Build history of the part. All positions in model axes, mm. Face numbers are marked on the shaded views. A direction names the side the tool comes from. Coordinates: 2 decimals unless noted, no trailing zeros. Loops run counter-clockwise (first coordinate to the right, second up) from the corner with the lowest first, then second, coordinate; pieces in that order, holes last.
Item 1: Cut at C-C (x = -0.25). List the corners of the cut face in (y, z), and give its area (3 significant figures).
Item 2: Drill centre lines: line 1 along X through (y, z) = (-0.25, 4); line 2 along Y through (x, z) = (8.48, 3.75); line 3 along X through (y, z) = (-0.5, 2). Where is each one in solid material? Low to high.
Item 3: Cut at A-A (z = 1.5). List the corners of the cut face in (x, y) (3 decimals), and give its area (3 significant figures).
Item 4: 3-axis set-ups, long thin cutter, end or side, ignore diameter. For the marked faces 1 and 2: which of +Z, -Z, +X, -X, +Y, -Y reach the whole face in a straight line?
Item 5: Flat gauge pin, fed straight in: pin 1 (4 mm diameter, centred on x = 3, y = 1, fed in from +Z). Where does the tip first touch, or does it go through?
Item 6: Cut at D-D (y = -2). List the corners of the cut face in (x, z), and give its area (3 significant figures).
Item 7: Cut at B-B (y = 0). List the corners of the cut face in (x, z).
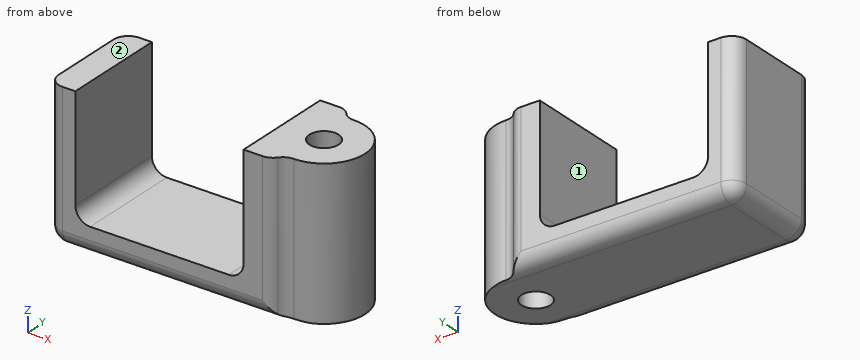
from build123d import *

# Parameters (mm, degrees)
F0_W         = 1.85
F0_H         = 7
F0_W_2       = 11.3
F1_DEPTH     = 1.85
F2_DEPTH     = 8
F3_T1_DEPTH  = 9.85
F3_T3_DEPTH  = 9.85
F3_T5_DEPTH  = 7
F3_T7_DEPTH  = 7
F3_T9_DEPTH  = 12
F4_T1_DEPTH  = 11.35
F4_T3_DEPTH  = 16.5
F4_T5_DEPTH  = 12.8150682373
F4_T8_ANGLE  = 90.0000000053
F4_T10_ANGLE = 90.0000000053


# Not quite as in the source:
# - a fillet or chamfer that OpenCascade refuses, or shapes differently, is made with other operations: its cross-section is extruded or revolved along the edge and cut away or added


with BuildPart() as f1:
    # F0 (on Top) → F1 (new body)
    with BuildSketch(Plane.XY):
        with Locations((-6.575, 0)):
            Rectangle(F0_W, F0_H)
        Rectangle(F0_W_2, F0_H)
        with BuildLine():
            Line((7.5, 0), (7.5, 2.5694551952))
            ThreePointArc((7.5, 2.5694551952), (5.73, 0), (7.5, -2.5694551952))
            Line((7.5, -2.5694551952), (7.5, 0))
        make_face()
        with BuildLine():
            Line((7.5, 2.5694551952), (7.5, 3.5))
            Line((7.5, 3.5), (5.65, 3.5))
            Line((5.65, 3.5), (5.65, -3.5))
            Line((5.65, -3.5), (7.5, -3.5))
            Line((7.5, -3.5), (7.5, -2.5694551952))
            ThreePointArc((7.5, -2.5694551952), (5.73, 0), (7.5, 2.5694551952))
        make_face()
        with BuildLine():
            ThreePointArc((11.23, 0), (10.0400480762, 2.2646743695), (7.5, 2.5694551952))
            Line((7.5, 2.5694551952), (7.5, 0))
            Line((7.5, 0), (7.5, -2.5694551952))
            ThreePointArc((7.5, -2.5694551952), (10.0400480762, -2.2646743695), (11.23, 0))
        make_face()
        with BuildLine():
            ThreePointArc((9.46, 0), (8.48, -0.98), (7.5, 0))
            ThreePointArc((7.5, 0), (8.48, 0.98), (9.46, 0))
        make_face(mode=Mode.SUBTRACT)
    extrude(amount=-F1_DEPTH)

    # F0 (on Top) → F2 (join)
    with BuildSketch(Plane.XY):
        with Locations((-6.575, 0)):
            Rectangle(F0_W, F0_H)
        with BuildLine():
            Line((7.5, 2.5694551952), (7.5, 3.5))
            Line((7.5, 3.5), (5.65, 3.5))
            Line((5.65, 3.5), (5.65, -3.5))
            Line((5.65, -3.5), (7.5, -3.5))
            Line((7.5, -3.5), (7.5, -2.5694551952))
            ThreePointArc((7.5, -2.5694551952), (5.73, 0), (7.5, 2.5694551952))
        make_face()
        with BuildLine():
            Line((7.5, 0), (7.5, 2.5694551952))
            ThreePointArc((7.5, 2.5694551952), (5.73, 0), (7.5, -2.5694551952))
            Line((7.5, -2.5694551952), (7.5, 0))
        make_face()
        with BuildLine():
            ThreePointArc((11.23, 0), (10.0400480762, 2.2646743695), (7.5, 2.5694551952))
            Line((7.5, 2.5694551952), (7.5, 0))
            Line((7.5, 0), (7.5, -2.5694551952))
            ThreePointArc((7.5, -2.5694551952), (10.0400480762, -2.2646743695), (11.23, 0))
        make_face()
        with BuildLine():
            ThreePointArc((9.46, 0), (8.48, -0.98), (7.5, 0))
            ThreePointArc((7.5, 0), (8.48, 0.98), (9.46, 0))
        make_face(mode=Mode.SUBTRACT)
    extrude(amount=F2_DEPTH)

    # F3: fillet of radius 1 on 5 edges, made by hand

    # F3_s2 → F3_t1 (join)
    with BuildSketch(Plane.XY.offset(-1.85)):
        with BuildLine():
            ThreePointArc((7.5, 3.5), (7.8571098794, 2.9584596209), (8.4713837652, 2.7499865019))
            ThreePointArc((8.4713837652, 2.7499865019), (7.9775177584, 2.7037033116), (7.5, 2.5694551952))
            Line((7.5, 2.5694551952), (7.5, 3.5))
        make_face()
    extrude(amount=F3_T1_DEPTH)

    # F3_s4 → F3_t3 (join)
    with BuildSketch(Plane.XY.offset(-1.85)):
        with BuildLine():
            ThreePointArc((7.5, -3.5), (7.8571098794, -2.9584596209), (8.4713837652, -2.7499865019))
            ThreePointArc((8.4713837652, -2.7499865019), (7.9775177584, -2.7037033116), (7.5, -2.5694551952))
            Line((7.5, -2.5694551952), (7.5, -3.5))
        make_face()
    extrude(amount=F3_T3_DEPTH)

    # F3_s6 → F3_t5 (join)
    with BuildSketch(Plane.XZ.offset(-3.5)):
        with BuildLine():
            ThreePointArc((5.65, 1), (5.3571067812, 0.2928932188), (4.65, 0))
            Line((4.65, 0), (5.65, 0))
            Line((5.65, 0), (5.65, 1))
        make_face()
    extrude(amount=F3_T5_DEPTH)

    # F3_s8 → F3_t7 (join)
    with BuildSketch(Plane.XZ.offset(-3.5)):
        with BuildLine():
            ThreePointArc((-4.65, 0), (-5.3571067812, 0.2928932188), (-5.65, 1))
            Line((-5.65, 1), (-5.65, 0))
            Line((-5.65, 0), (-4.65, 0))
        make_face()
    extrude(amount=F3_T7_DEPTH)

    # F3_s10 → F3_t9 (cut)
    with BuildSketch(Plane.XZ.offset(-6)):
        with BuildLine():
            ThreePointArc((-7.5, -0.85), (-7.2071067812, -1.5571067812), (-6.5, -1.85))
            Line((-6.5, -1.85), (-7.5, -1.85))
            Line((-7.5, -1.85), (-7.5, -0.85))
        make_face()
    extrude(amount=F3_T9_DEPTH, mode=Mode.SUBTRACT)

    # F4: fillet of radius 1 on 8 edges, made by hand

    # F4_s2 → F4_t1 (cut)
    with BuildSketch(Plane.XY.offset(-0.85)):
        with BuildLine():
            ThreePointArc((-7.5, 2.5), (-7.2071067812, 3.2071067812), (-6.5, 3.5))
            Line((-6.5, 3.5), (-7.5, 3.5))
            Line((-7.5, 3.5), (-7.5, 2.5))
        make_face()
        with BuildLine():
            ThreePointArc((-7.5, -2.5), (-7.2071067812, -3.2071067812), (-6.5, -3.5))
            Line((-6.5, -3.5), (-7.5, -3.5))
            Line((-7.5, -3.5), (-7.5, -2.5))
        make_face()
    extrude(amount=F4_T1_DEPTH, mode=Mode.SUBTRACT)

    # F4_s4 → F4_t3 (cut)
    with BuildSketch(Plane.YZ.offset(-6.5)):
        with BuildLine():
            ThreePointArc((3.5, -0.85), (3.2071067812, -1.5571067812), (2.5, -1.85))
            Line((2.5, -1.85), (3.5, -1.85))
            Line((3.5, -1.85), (3.5, -0.85))
        make_face()
        with BuildLine():
            ThreePointArc((-3.5, -0.85), (-3.2071067812, -1.5571067812), (-2.5, -1.85))
            Line((-2.5, -1.85), (-3.5, -1.85))
            Line((-3.5, -1.85), (-3.5, -0.85))
        make_face()
    extrude(amount=F4_T3_DEPTH, mode=Mode.SUBTRACT)

    # F4_s6 → F4_t5 (cut)
    with BuildSketch(Plane.XY.offset(-3.3325341187)):
        with BuildLine():
            ThreePointArc((6.9069863525, 3.5), (7.3400043679, 3.4013852663), (7.6876184707, 3.1249907968))
            ThreePointArc((7.6876184707, 3.1249907968), (7.5739320459, 3.3025507681), (7.5, 3.5))
            Line((7.5, 3.5), (6.9069863525, 3.5))
        make_face()
        with BuildLine():
            ThreePointArc((6.9069863525, -3.5), (7.3400043679, -3.4013852663), (7.6876184707, -3.1249907968))
            ThreePointArc((7.6876184707, -3.1249907968), (7.5739320459, -3.3025507681), (7.5, -3.5))
            Line((7.5, -3.5), (6.9069863525, -3.5))
        make_face()
    extrude(amount=F4_T5_DEPTH, mode=Mode.SUBTRACT)

    # F4_s7 → F4_t8 (revolve, cut)
    with BuildSketch(Plane.YZ.offset(-6.5)):
        with BuildLine():
            ThreePointArc((3.5, -0.85), (3.2071067812, -1.5571067812), (2.5, -1.85))
            Line((2.5, -1.85), (3.5, -1.85))
            Line((3.5, -1.85), (3.5, -0.85))
        make_face()
    revolve(axis=Axis((-6.5, 3.5, -0.85), (0, 1, 0)), revolution_arc=F4_T8_ANGLE, mode=Mode.SUBTRACT)

    # F4_s9 → F4_t10 (revolve, cut)
    with BuildSketch(Plane.YZ.offset(-6.5)):
        with BuildLine():
            ThreePointArc((-3.5, -0.85), (-3.2071067812, -1.5571067812), (-2.5, -1.85))
            Line((-2.5, -1.85), (-3.5, -1.85))
            Line((-3.5, -1.85), (-3.5, -0.85))
        make_face()
    revolve(axis=Axis((-6.5, -3.5, -0.85), (0, 1, 0)), revolution_arc=F4_T10_ANGLE, mode=Mode.SUBTRACT)


solid = f1.part
Filled sheet:
1. outline: (-3.5, -0.85) arc R1 ccw to (-2.5, -1.85) - (2.5, -1.85) arc R1 ccw to (3.5, -0.85) - (3.5, 0) - (-3.5, 0) - close
1. area: 12.5 mm2
2. line 1: x = -7.5 to -5.65, 5.65 to 7.53, 9.43 to 11.22
2. line 2: y = -2.75 to -0.98, 0.98 to 2.75
2. line 3: x = -7.5 to -5.65, 5.65 to 7.64, 9.32 to 11.18
3. outline: (-7.5, -2.5) arc R1 ccw to (-6.5, -3.5) - (-5.65, -3.5) - (-5.65, 3.5) - (-6.5, 3.5) arc R1 ccw to (-7.5, 2.5) - close; (5.65, -3.5) - (6.907, -3.5) arc R1 ccw to (7.688, -3.125) arc R1 cw to (8.471, -2.75) arc R2.75 ccw (long way) to (8.471, 2.75) arc R1 cw to (7.688, 3.125) arc R1 ccw to (6.907, 3.5) - (5.65, 3.5) - close; hole circle Ø1.96 at (8.48, 0)
3. area: 40.0 mm2
4. face 1: +Z, +Y, -Y
4. face 2: +Z, +X, -X, +Y, -Y
5. pin 1: stops at z = 0.06
6. outline: (-7.5, -0.85) arc R1 ccw to (-6.5, -1.85) - (10.37, -1.85) - (10.37, 8) - (5.65, 8) - (5.65, 1) arc R1 cw to (4.65, 0) - (-4.65, 0) arc R1 cw to (-5.65, 1) - (-5.65, 8) - (-7.5, 8) - close
6. area: 85.8 mm2
7. outline: (-7.5, -0.85) arc R1 ccw to (-6.5, -1.85) - (7.5, -1.85) - (7.5, 8) - (5.65, 8) - (5.65, 1) arc R1 cw to (4.65, 0) - (-4.65, 0) arc R1 cw to (-5.65, 1) - (-5.65, 8) - (-7.5, 8) - close; (9.46, -1.85) - (11.23, -1.85) - (11.23, 8) - (9.46, 8) - close
